Part model, mm, in its own coordinate system. Give positions to 0.01 mm unless a question says otherwise; leave off trailing zeros. Order: outer loops, then holes, each group sorted by start corner. A loop starts at its lowest first (then second) coordinate and runs counter-clockwise, first axis right, second up.
1. Slice it at B-B on z = 60. List the corners of the cut face in (x, y).
2. Drop flat-ended pins along their axis: pin 1 Ø1.5 at (y, z) = (2.5, -40.5) entering from -X; pin 2 Ø4 at (x, z) = (1, -39.5) entering from +Y; pin 3 Ø0.5 at (x, y) = (-0.5, 3.5) entering from -Z. Give the stop position or say it passes through.
3. Probe line 1 (Z direction, x = -0.25, y = 3.5); line 2 (X direction, y = -3, z = -45.5); line 3 (X direction, y = 1.5, z = 10). List the from-to ranges inside material, lowest first.
4. Slice it at C-C on y = -1.25. List the corners of the cut face in (x, z), and give its area (3 significant figures).
5. Slice it at A-A on x = 0. List the corners of the cut face in (y, z), and give its area (3 significant figures).
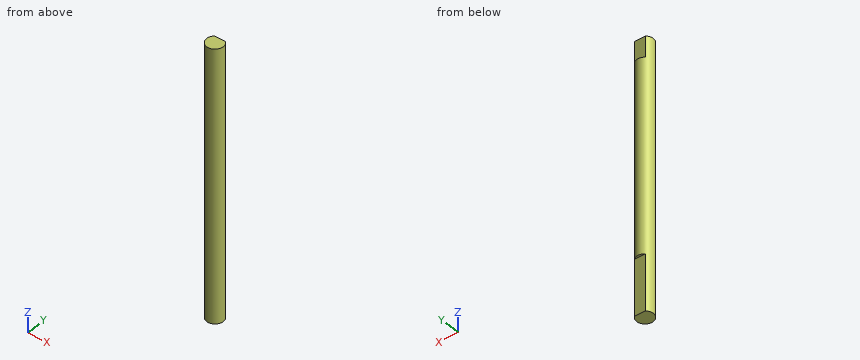
from build123d import *

# Parameters (mm, degrees)
ESBO_O1_R                     = 4
RESSALTO_EXTRUS_O1_DEPTH      = 72
RESSALTO_EXTRUS_O1_DEPTH_BACK = 58
CORTE_EXTRUS_O1_DEPTH         = 10
CORTE_EXTRUS_O2_DEPTH         = 27


with BuildPart() as part:
    # Esboço1 → Ressalto-extrusão1 (new body, two sides)
    with BuildSketch(Plane.XY) as ressalto_extrus_o1_sk:
        Circle(ESBO_O1_R)
    extrude(amount=RESSALTO_EXTRUS_O1_DEPTH)
    extrude(ressalto_extrus_o1_sk.sketch, amount=-RESSALTO_EXTRUS_O1_DEPTH_BACK)

    # Esboço2 → Corte-extrusão1 (cut)
    with BuildSketch(Plane.XY.offset(72)):
        with BuildLine():
            Line((2.645751311, 3), (-2.645751311, 3))
            ThreePointArc((-2.645751311, 3), (0, 4), (2.645751311, 3))
        make_face()
    extrude(amount=-CORTE_EXTRUS_O1_DEPTH, mode=Mode.SUBTRACT)

    # Esboço6 → Corte-extrusão2 (cut)
    with BuildSketch(Plane(origin=(0, 0, -58), x_dir=(-1, 0, 0), z_dir=(0, 0, -1))):
        with BuildLine():
            Line((2.645751311, 3), (-2.645751311, 3))
            ThreePointArc((-2.645751311, 3), (0, 4), (2.645751311, 3))
        make_face()
    extrude(amount=-CORTE_EXTRUS_O2_DEPTH, mode=Mode.SUBTRACT)


solid = part.part
Data:
1. outline: circle Ø8 at (0, 0)
2. pin 1: stops at x = -3.6
2. pin 2: stops at y = 3
2. pin 3: stops at z = -31
3. line 1: z = -31 to 62
3. line 2: x = -2.65 to 2.65
3. line 3: x = -3.71 to 3.71
4. outline: (-3.8, -58) - (3.8, -58) - (3.8, 72) - (-3.8, 72) - close
4. area: 988 mm2
5. outline: (-4, -58) - (3, -58) - (3, -31) - (4, -31) - (4, 62) - (3, 62) - (3, 72) - (-4, 72) - close
5. area: 1,000 mm2
